Geometry: final body of the model. Coordinates: model frame, mm. A direction names the side the tool comes from. Give positions to 0.01 mm unless a question says otherwise; leave off trailing zeros. Write each loop counter-clockwise with the first axis right and the second up, starting at its lowest first coordinate (ties: lowest second). Pieces come first, ordered by that corner, then holes. Notation, with made-up numbers: M -11.5,6.25 L 7.5,6.25 A21 ccw 7.5,31.25 Z; hole C 46.25,-2.5 d5. An arc over 180 degrees is marked long. Use a Markdown table: item, result. Add a question column.
1) Section C-C on z = 30.5. Return the cut outline in (x, y).
2) Draft query along Y for faces 3 (the cylindrical face through (40.287, 46.767, 4.918)), 4 (the flat face through (16, 1, 10)), 5 (the cylindrical face through (6.466, -2.681, 50.278)). Return one class per face: +Y half, -Y half, draft (parallel to the pull), parting line (faces both ways), or undercut.
3) Section D-D on y = 65.5. Return the cut outline in (x, z), then the cut area to 3 significant figures.
4) Set-up query: faces 1 (the cylindrical face through (-19.642, -58.273, 4.918)), 2 (the flat face through (-13, 10, 7)). Return all of +Z, -Z, +X, -X, +Y, -Y with unobstructed straight access to the full face (end or side cutting, diameter ignored); none if empty.
5) Line query: line 1 (X direction, y = 8, z = 3); line 2 (X direction, y = 8.25, z = 9.4); line 3 (Z direction, x = 50.5, y = 10). Output: solid intervals per line, ascending.
6) Section A-A on y = -61. Return the cut outline in (x, z) (3 decimals).
7) Section B-B on x = -20. Return the cut outline in (y, z) (3 decimals), then the cut area to 3 significant figures.
8) Pin query (flat end, axial travel): pin 1 (4 mm diameter, centred on x = -46, z = 11.5, fed in from -Y); pin 2 (6.5 mm diameter, centred on x = -42.83, y = 47.82, fed in from +Z); pin 3 (9 mm diameter, centred on x = 1, z = 84, fed in from +Y). Return the tip coordinate at first contact, or that it passes through.
```python
from build123d import *

# Parameters (mm, degrees)
SKETCH1_R                      = 78
BOSS_EXTRUDE1_DEPTH            = 10
CBORE_FOR_M3_SHCS1_AT_2_COUNT  = 2
CBORE_FOR_M3_SHCS1_AT_2_PITCH  = 28.578838325
CBORE_FOR_M3_SHCS1_AT_3_COUNT  = 2
CBORE_FOR_M3_SHCS1_AT_3_PITCH  = 28.578838325
SKETCH6_R                      = 7
BOSS_EXTRUDE2_DEPTH            = 81.7
SKETCH20_W                     = 8
SKETCH20_H                     = 8
CUT_EXTRUDE1_DEPTH             = 20
M5_CLEARANCE_HOLE3_D           = 5.5
M5_CLEARANCE_HOLE3_CSINK_D     = 5.55
M5_CLEARANCE_HOLE3_CSINK_ANGLE = 90
CIRPATTERN1_COUNT              = 3
M3_CLEARANCE_HOLE2_D           = 3.4
M3_CLEARANCE_HOLE2_CSINK_D     = 3.45
M3_CLEARANCE_HOLE2_CSINK_ANGLE = 90


with BuildPart() as part:
    # Sketch1 → Boss-Extrude1 (new body)
    with BuildSketch(Plane.XY):
        Circle(SKETCH1_R)
    extrude(amount=BOSS_EXTRUDE1_DEPTH)

    # Sketch4 → CBORE for M3 SHCS1 (revolve, cut)
    with BuildSketch(Plane(origin=(-14.289419162, 8.25, 10), x_dir=(0, -1, 0), z_dir=(1, 0, 0))):
        Polygon((0, 0), (0, 10), (1.7, 10), (1.7, 3), (3.25, 3), (3.25, 0.025), (3.275, 0), align=None)
    cbore_for_m3_shcs1 = revolve(axis=Axis((-14.289419162, 8.25, 16.35), (0, 0, -1)), mode=Mode.SUBTRACT)

    # CBORE for M3 SHCS1 at 2: CBORE for M3 SHCS1 ×2
    with Locations(*[(i * CBORE_FOR_M3_SHCS1_AT_2_PITCH, 0, 0) for i in range(1, CBORE_FOR_M3_SHCS1_AT_2_COUNT)]):
        add(cbore_for_m3_shcs1, mode=Mode.SUBTRACT)

    # CBORE for M3 SHCS1 at 3: CBORE for M3 SHCS1 ×2
    with Locations(*[Vector(0.5000000000000012, -0.866025403784438, 0) * (i * CBORE_FOR_M3_SHCS1_AT_3_PITCH) for i in range(1, CBORE_FOR_M3_SHCS1_AT_3_COUNT)]):
        add(cbore_for_m3_shcs1, mode=Mode.SUBTRACT)

    # Sketch6 → Boss-Extrude2 (add)
    with BuildSketch(Plane.XY.offset(10)):
        Circle(SKETCH6_R)
    extrude(amount=BOSS_EXTRUDE2_DEPTH)

    # Sketch20 → Cut-Extrude1 (cut)
    with BuildSketch(Plane.XY.offset(91.7)):
        Rectangle(SKETCH20_W, SKETCH20_H)
    extrude(amount=-CUT_EXTRUDE1_DEPTH, mode=Mode.SUBTRACT)

    # M5 Clearance Hole3 (through all)
    with Locations(Plane.XY.offset(10)):
        with Locations((-20, -61), (20, -61)):
            m5_clearance_hole3 = CounterSinkHole(M5_CLEARANCE_HOLE3_D / 2, M5_CLEARANCE_HOLE3_CSINK_D / 2, counter_sink_angle=M5_CLEARANCE_HOLE3_CSINK_ANGLE)

    # CirPattern1: M5 Clearance Hole3 ×3 about axis
    cirpattern1_axis = Axis((0, 0, 0), (0, 0, 1))
    for i in range(1, CIRPATTERN1_COUNT):
        add(m5_clearance_hole3.rotate(cirpattern1_axis, i * 360 / CIRPATTERN1_COUNT), mode=Mode.SUBTRACT)

    # M3 Clearance Hole2 (through all)
    with Locations(Plane(origin=(7, 0, 0), x_dir=(0, 0, -1), z_dir=(1, 0, 0))):
        with Locations((-81.7, 0)):
            CounterSinkHole(M3_CLEARANCE_HOLE2_D / 2, M3_CLEARANCE_HOLE2_CSINK_D / 2, counter_sink_angle=M3_CLEARANCE_HOLE2_CSINK_ANGLE)


solid = part.part
```
Found:
| question | item | result |
|---|---|---|
| 1 | outline | C 0,0 d14 |
| 2 | face 3 | undercut |
| 2 | face 4 | draft |
| 2 | face 5 | parting line |
| 3 | outline | M -42.35,0 L 42.35,0 L 42.35,10 L -42.35,10 Z |
| 3 | area | 847 mm² |
| 4 | face 1 | +Z, -Z |
| 4 | face 2 | +Z |
| 5 | line 1 | -77.59 to -15.97, -12.61 to 12.61, 15.97 to 77.59 |
| 5 | line 2 | -77.56 to -17.54, -11.04 to 11.04, 17.54 to 77.56 |
| 5 | line 3 | 0 to 10 |
| 6 | outline | M -48.611,0 L -22.75,0 L -22.75,9.975 L -22.775,10 L -48.611,10 Z; M -17.25,0 L 17.25,0 L 17.25,9.975 L 17.225,10 L -17.225,10 L -17.25,9.975 Z; M 22.75,0 L 48.611,0 L 48.611,10 L 22.775,10 L 22.75,9.975 Z |
| 7 | outline | M -75.392,0 L -63.75,0 L -63.75,9.975 L -63.775,10 L -75.392,10 Z; M -58.25,0 L 75.392,0 L 75.392,10 L -58.225,10 L -58.25,9.975 Z |
| 7 | area | 1,450 mm² |
| 8 | pin 1 | y = -63.94 |
| 8 | pin 2 | z = 10 |
| 8 | pin 3 | y = 7 |
